from build123d import *

# Parameters (mm, degrees)
SKETCH_1_W      = 90
SKETCH_1_H      = 62.5
SKETCH_1_R      = 1.6
SKETCH_1_R_2    = 2.15
SKETCH_1_R_3    = 2.6
SKETCH_1_W_2    = 70
SKETCH_1_H_2    = 31
EXTRUDE_1_DEPTH = 3
FILLET_1_R      = 5
FILLET_2_R      = 2


with BuildPart() as part:
    # ｽｹｯﾁ1 → ﾎﾞｽ - 押し出し1 (new body)
    with BuildSketch(Plane.XY):
        with Locations((0, 5.75)):
            Rectangle(SKETCH_1_W, SKETCH_1_H)
        with Locations((40, 20.5)):
            Circle(SKETCH_1_R, mode=Mode.SUBTRACT)
        with Locations((40, 32)):
            Circle(SKETCH_1_R_2, mode=Mode.SUBTRACT)
        with Locations(Location((-40, 32, 0), (0, 0, 180))):
            Circle(SKETCH_1_R_2, mode=Mode.SUBTRACT)
        with Locations(Location((40, -20.5, 0), (0, 0, 180))):
            Circle(SKETCH_1_R, mode=Mode.SUBTRACT)
        with Locations(Location((-40, 20.5, 0), (0, 0, 180))):
            Circle(SKETCH_1_R, mode=Mode.SUBTRACT)
        with Locations((-40, -20.5)):
            Circle(SKETCH_1_R, mode=Mode.SUBTRACT)
        with Locations((0, 32)):
            Circle(SKETCH_1_R_3, mode=Mode.SUBTRACT)
        Rectangle(SKETCH_1_W_2, SKETCH_1_H_2, mode=Mode.SUBTRACT)
    extrude(amount=EXTRUDE_1_DEPTH)

    # ﾌｨﾚｯﾄ1
    fillet_1_edges = [part.edges().sort_by_distance(p)[0] for p in [
        (-35, 15.5, 1.5),
        (-35, -15.5, 1.5),
        (35, -15.5, 1.5),
        (35, 15.5, 1.5),
    ]]
    fillet(fillet_1_edges, radius=FILLET_1_R)

    # ﾌｨﾚｯﾄ2
    fillet_2_edges = [part.edges().sort_by_distance(p)[0] for p in [
        (45, -25.5, 1.5),
        (-45, -25.5, 1.5),
        (-45, 37, 1.5),
        (45, 37, 1.5),
    ]]
    fillet(fillet_2_edges, radius=FILLET_2_R)


solid = part.part
Part model, mm, in its own coordinate system. A direction names the side the tool comes from. Coordinates: 2 decimals unless noted, no trailing zeros. Order: outer loops, then holes, each group sorted by start corner. A loop starts at its lowest first (then second) coordinate and runs counter-clockwise, first axis right, second up.
(1) Probe L1, parallel to Y at x = 0, z = 1.1; L2, parallel to Y at x = 40, z = 1.5; L3, parallel to X at y = -7, z = 1.7. List the from-to ranges inside material, lowest first.
Check sheet entries:
L1: y = -25.5 to -15.5, 15.5 to 29.4, 34.6 to 37
L2: y = -25.5 to -22.1, -18.9 to 18.9, 22.1 to 29.85, 34.15 to 37
L3: x = -45 to -35, 35 to 45
(2) Slice it at A-A, the plane x = 40. Write the cut outline in (y, z).
Check sheet entries:
outline: (-25.5, 0) - (-22.1, 0) - (-22.1, 3) - (-25.5, 3) - close; (-18.9, 0) - (18.9, 0) - (18.9, 3) - (-18.9, 3) - close; (22.1, 0) - (29.85, 0) - (29.85, 3) - (22.1, 3) - close; (34.15, 0) - (37, 0) - (37, 3) - (34.15, 3) - close
(3) Pin check, flat tips, straight feed: pin 1 Ø2.5 at (x, y) = (-40, 32) entering from +Z; pin 2 Ø5 at (x, y) = (40, -20.5) entering from -Z. Stop position of each tip, or through.
Check sheet entries:
pin 1: passes through
pin 2: stops at z = 0
(4) Slice it at D-D, the plane y = -6. Write the cut outline in (x, z).
Check sheet entries:
outline: (-45, 0) - (-35, 0) - (-35, 3) - (-45, 3) - close; (35, 0) - (45, 0) - (45, 3) - (35, 3) - close
(5) Pull direction Y, two halves, no side cores. Call faces 3 (the face through (44.4, -24.93, 1.52)), 4 (the face through (44.4, 36.43, 1.52)), 5 (the face through (-45, 5, 1)), 6 (the face through (33.5, -14.07, 1.52)): pulls with the +Y half, pulls with the -Y half, needs draft (parallel to the pull), parting line crosses it, or undercut.
Check sheet entries:
face 3: pulls with the -Y half
face 4: pulls with the +Y half
face 5: needs draft
face 6: undercut
(6) Slice it at C-C, the plane x = -16. Write the cut outline in (y, z).
Check sheet entries:
outline: (-25.5, 0) - (-15.5, 0) - (-15.5, 3) - (-25.5, 3) - close; (15.5, 0) - (37, 0) - (37, 3) - (15.5, 3) - close
(7) Slice it at B-B, the plane y = 32. Write the cut outline in (x, z).
Check sheet entries:
outline: (-45, 0) - (-42.15, 0) - (-42.15, 3) - (-45, 3) - close; (-37.85, 0) - (-2.6, 0) - (-2.6, 3) - (-37.85, 3) - close; (2.6, 0) - (37.85, 0) - (37.85, 3) - (2.6, 3) - close; (42.15, 0) - (45, 0) - (45, 3) - (42.15, 3) - close
(8) Tool access for faces 1 (the face through (-1, 20, 3)), 2 (the face through (0, 15.5, 1)): list every direction of +Z, -Z, +X, -X, +Y, -Y with a clear straight run to the whole face (end or side of a thin tool).
Check sheet entries:
face 1: +Z, +X, -X, +Y, -Y
face 2: +Z, -Z
